Source: CAD feature listing. Evaluate the final solid. Frame: model axes, mm. A direction names the side the tool comes from. Round coordinates to 2 decimals unless told otherwise and drop trailing zeros. Order: outer loops, then holes, each group sorted by start corner. A loop starts at its lowest first (then second) coordinate and runs counter-clockwise, first axis right, second up. Notation, with made-up numbers: (17.5, 26.5) -> (40.5, 26.5) arc R13 cw to (40.5, 46.5) -> close; hole circle Ø11 at (-35, -13.5). An arc over 180 degrees is marked (long way). Answer as CSV lines item,"result".
from build123d import *

# Parameters (mm, degrees)
F0_R     = 26
F0_R_2   = 10.85
F1_DEPTH = 6.67
F2_SIZE  = 0.2
F3_R     = 16
F4_DEPTH = 6.2
F5_R     = 10.85
F6_DEPTH = 11


with BuildPart() as f1:
    # F0 (on Front) → F1 (new body)
    with BuildSketch(Plane.XZ):
        Circle(F0_R)
        with BuildLine():
            ThreePointArc((-2.5914037581, -15.78875), (0, -13.4), (2.5914037581, -15.78875))
            Line((2.5914037581, -15.78875), (2.5914037581, -17.2977615707))
            ThreePointArc((2.5914037581, -17.2977615707), (-0.0087763318, -20.1007524005), (-2.5914037581, -17.2815805949))
            Line((-2.5914037581, -17.2815805949), (-2.5914037581, -15.78875))
        make_face(mode=Mode.SUBTRACT)
        with BuildLine():
            ThreePointArc((15.78875, -2.5914037581), (13.4, 0), (15.78875, 2.5914037581))
            Line((15.78875, 2.5914037581), (17.3070686878, 2.5914037581))
            ThreePointArc((17.3070686878, 2.5914037581), (20.1000462874, -0.0189616291), (17.2721013057, -2.5914037581))
            Line((17.2721013057, -2.5914037581), (15.78875, -2.5914037581))
        make_face(mode=Mode.SUBTRACT)
        with BuildLine():
            ThreePointArc((-17.3068571429, -2.592816198), (-20.1, 0), (-17.3068571429, 2.592816198))
            Line((-17.3068571429, 2.592816198), (-16.014371015, 2.5999602831))
            ThreePointArc((-16.014371015, 2.5999602831), (-13.4, 0), (-16.014371015, -2.5999602831))
            Line((-16.014371015, -2.5999602831), (-17.3068571429, -2.592816198))
        make_face(mode=Mode.SUBTRACT)
        Circle(F0_R_2, mode=Mode.SUBTRACT)
        with BuildLine():
            ThreePointArc((2.5914037581, 15.78875), (0, 13.4), (-2.5914037581, 15.78875))
            Line((-2.5914037581, 15.78875), (-2.5914037581, 17.2976958265))
            ThreePointArc((-2.5914037581, 17.2976958265), (-0.0037683158, 20.0993370021), (2.5936213204, 17.3067365048))
            Line((2.5936213204, 17.3067365048), (2.5936213204, 15.8179877846))
            Line((2.5936213204, 15.8179877846), (2.5936213204, 15.78875))
            Line((2.5936213204, 15.78875), (2.5914037581, 15.78875))
        make_face(mode=Mode.SUBTRACT)
    extrude(amount=-F1_DEPTH)

    # F2
    f2_edges = [f1.edges().sort_by_distance(p)[0] for p in [
        (-26, 6.67, 0),
        (-26, 0, 0),
    ]]
    chamfer(f2_edges, length=F2_SIZE)

    # F3 (on face) → F4 (join)
    with BuildSketch(Plane.XZ):
        Circle(F3_R)
    extrude(amount=F4_DEPTH)

    # F5 (on face) → F6 (cut)
    with BuildSketch(Plane.XZ.offset(6.2)):
        Circle(F5_R)
        with BuildLine():
            Line((3.4739061675, 14.57341362), (3.4833905794, 18.1594268488))
            ThreePointArc((3.4833905794, 18.1594268488), (0.0005451634, 21.9999999575), (-3.4834965064, 18.1605120179))
            Line((-3.4834965064, 18.1605120179), (-3.4760989469, 14.5916666667))
            ThreePointArc((-3.4760989469, 14.5916666667), (-0.0091921433, 11.5000120708), (3.4739061675, 14.57341362))
        make_face()
        with BuildLine():
            Line((-14.57341362, 3.4739061675), (-18.1594268488, 3.4833905794))
            ThreePointArc((-18.1594268488, 3.4833905794), (-21.9999999575, 0.0005451634), (-18.1605120179, -3.4834965064))
            Line((-18.1605120179, -3.4834965064), (-14.5916666667, -3.4760989469))
            ThreePointArc((-14.5916666667, -3.4760989469), (-11.5000120708, -0.0091921433), (-14.57341362, 3.4739061675))
        make_face()
        with BuildLine():
            Line((-3.4739061675, -14.57341362), (-3.4833905794, -18.1594268488))
            ThreePointArc((-3.4833905794, -18.1594268488), (-0.0005451634, -21.9999999575), (3.4834965064, -18.1605120179))
            Line((3.4834965064, -18.1605120179), (3.4760989469, -14.5916666667))
            ThreePointArc((3.4760989469, -14.5916666667), (0.0091921433, -11.5000120708), (-3.4739061675, -14.57341362))
        make_face()
        with BuildLine():
            Line((14.57341362, -3.4739061675), (18.1594268488, -3.4833905794))
            ThreePointArc((18.1594268488, -3.4833905794), (21.9999999575, -0.0005451634), (18.1605120179, 3.4834965064))
            Line((18.1605120179, 3.4834965064), (14.5916666667, 3.4760989469))
            ThreePointArc((14.5916666667, 3.4760989469), (11.5000120708, 0.0091921433), (14.57341362, -3.4739061675))
        make_face()
    extrude(amount=-F6_DEPTH, mode=Mode.SUBTRACT)


solid = f1.part
1. Section query B-B on x = 0. Return loops of the section in (y, z).
Results below:
outline,"(-6.2, -11.5) -> (4.8, -11.5) -> (4.8, -13.4) -> (6.67, -13.4) -> (6.67, -10.85) -> (-6.2, -10.85) -> close; (-6.2, 10.85) -> (6.67, 10.85) -> (6.67, 13.4) -> (4.8, 13.4) -> (4.8, 11.5) -> (-6.2, 11.5) -> close; (0, -25.8) -> (0.2, -26) -> (6.47, -26) -> (6.67, -25.8) -> (6.67, -20.1) -> (4.8, -20.1) -> (4.8, -22) -> (0, -22) -> close; (0, 22) -> (4.8, 22) -> (4.8, 20.1) -> (6.67, 20.1) -> (6.67, 25.8) -> (6.47, 26) -> (0.2, 26) -> (0, 25.8) -> close"
2. Pin query (flat end, axial travel): pin 1 (17.5 mm diameter, centred on x = 0, z = 0, fed in from +Y); pin 2 (3 mm diameter, centred on x = -19, y = 3.5, fed in from -Z); pin 3 (3 mm diameter, centred on x = 2.5, y = 2.5, fed in from -Z); pin 4 (0.8 mm diameter, centred on x = 16.5, y = 5.5, fed in from -Z). Return the tip coordinate at first contact, or that it passes through.
Results below:
pin 1,"through"
pin 2,"z = -19.23"
pin 3,"z = -25.98"
pin 4,"z = -20.42"
3. Section query A-A on z = 0. Return loops of the section in (x, y).
Results below:
outline,"(-26, 0.2) -> (-25.8, 0) -> (-22, 0) -> (-22, 4.8) -> (-20.1, 4.8) -> (-20.1, 6.67) -> (-25.8, 6.67) -> (-26, 6.47) -> close; (-13.4, 4.8) -> (-11.5, 4.8) -> (-11.5, -6.2) -> (-10.85, -6.2) -> (-10.85, 6.67) -> (-13.4, 6.67) -> close; (10.85, -6.2) -> (11.5, -6.2) -> (11.5, 4.8) -> (13.4, 4.8) -> (13.4, 6.67) -> (10.85, 6.67) -> close; (20.1, 4.8) -> (22, 4.8) -> (22, 0) -> (25.8, 0) -> (26, 0.2) -> (26, 6.47) -> (25.8, 6.67) -> (20.1, 6.67) -> close"
4. Mould query, pull axis Z, two halves, no side actions, for faces 1 (the cylindrical face through (11.402, -3.057, 11.224)), 2 (the flat face through (2.591, 6, -17)), 3 (the cylindrical face through (-11.402, -3.057, -11.224)), 4 (the cylindrical face through (-0.1, -0.8, 11.5)). Classes: released by +Z, released by -Z, zero draft, split by the parting line, or undercut.
Results below:
face 1,"released by +Z"
face 2,"undercut"
face 3,"released by -Z"
face 4,"undercut"
5. Line query: L1, parallel to Z at x = 0, y = 3.5; L2, parallel to Z at x = 0.5, y = 6; L3, parallel to X at y = 0.75, z = 1.5. Output: solid intervals per line, ascending. Write a range as [from, to].
Results below:
L1,"[-26, -22], [-11.5, -10.85], [10.85, 11.5], [22, 26]"
L2,"[-26, -20.05], [-13.45, -10.84], [10.84, 13.45], [20.05, 26]"
L3,"[-25.96, -21.66], [-11.84, -10.75], [10.75, 11.84], [21.66, 25.96]"
6. Reachability of faces 5 (the flat face through (17, 4.8, -3)), 6 (the cylindrical face through (11.224, -3.057, -11.402)), 7 (the flat face through (17, 6, -2.591)) from +Z, -Z, +X, -X, +Y, -Y: full face, straight path, thin tool, end or side. Return the list, or none.
Results below:
face 5,"-Y"
face 6,"-Z, +X, -Y"
face 7,"+Y, -Y"
7. Section query D-D on y = 3.75. Return loops of the section in (x, z), and give its area (3 significant figures).
Results below:
outline,"circle Ø52 at (0, 0); hole (-18.16, -3.48) -> (-14.59, -3.48) arc R3.5 ccw to (-14.57, 3.47) -> (-18.16, 3.48) arc R3.5 ccw (long way) to start; hole circle Ø21.7 at (0, 0); hole (-3.48, -18.16) arc R3.5 ccw (long way) to (3.48, -18.16) -> (3.48, -14.59) arc R3.5 ccw to (-3.47, -14.57) -> close; hole (-3.48, 14.59) arc R3.5 ccw to (3.47, 14.57) -> (3.48, 18.16) arc R3.5 ccw (long way) to (-3.48, 18.16) -> close; hole (14.57, -3.47) -> (18.16, -3.48) arc R3.5 ccw (long way) to (18.16, 3.48) -> (14.59, 3.48) arc R3.5 ccw to start"
area,"1,500 mm2"
8. Section query C-C on y = -1. Return loops of the section in (x, z), and give its area (3 significant figures).
Results below:
outline,"(-15.62, -3.48) arc R16 ccw to (-3.48, -15.62) -> (-3.47, -14.57) arc R3.5 cw to (3.48, -14.59) -> (3.48, -15.62) arc R16 ccw to (15.62, -3.48) -> (14.57, -3.47) arc R3.5 cw to (14.59, 3.48) -> (15.62, 3.48) arc R16 ccw to (3.48, 15.62) -> (3.47, 14.57) arc R3.5 cw to (-3.48, 14.59) -> (-3.48, 15.62) arc R16 ccw to (-15.62, 3.48) -> (-14.57, 3.47) arc R3.5 cw to (-14.59, -3.48) -> close; hole circle Ø21.7 at (0, 0)"
area,"333 mm2"
